The listing builds one solid part. Answer for the finished solid, in the listing's coordinates (mm). Give positions to 0.01 mm unless a question says otherwise; leave off trailing zeros. Loops run counter-clockwise (first coordinate to the right, second up) from the corner with the lowest first, then second, coordinate; pieces in that order, holes last. Notation, with made-up numbers: M 37,78 L 73,78 A15 cw 73,101 Z; hole C 70,-10 d11. An arc over 180 degrees is marked long. One line per item, written item: value. Start each with the question number.
Q1. A cutting plane is placed at B-B, the plane z = 9.5. Determine the outline of the cut face in (x, y), and give its area (3 significant figures).
Q2. Consider L1, parallel to Y at x = 1.25, z = 0; L2, parallel to Z at x = 0.2, y = 10; L3, parallel to Y at x = 0.3, z = -7. Determine where each line is inside the solid, lowest interval first.
Q3. A flat-ended cylindrical pin translates along its axis: pin 1 (5 mm diameter, centred on y = 95.25, z = 0, fed in from +X). Find the tip coordinate at first contact, or state that the pin passes through.
Q4. The mould has two halves that part along Z. Classify faces 1 (the cylindrical face through (0.783, 98.002, 1.755)), 2 (the cylindrical face through (0.78, 101.79, -4.5)), 3 (the flat face through (0, 45, 4)): +Z half, -Z half, draft (parallel to the pull), parting line (faces both ways), or undercut.
Q5. A cutting plane is placed at D-D, the plane y = 15. Determine the outline of the cut face in (x, z), and give its area (3 significant figures).
Q6. A cutting plane is placed at C-C, the plane x = 0.5. State how many separate pieces and enclosed holes the cut face has, and give its area (3 significant figures).
Q7. A cutting plane is placed at A-A, the plane z = 0. Determine the outline of the cut face in (x, y), and give its area (3 significant figures).
from build123d import *

# Parameters (mm, degrees)
SKETCH1_R               = 11.1125
BOSS_EXTRUDE1_DEPTH     = 1.5875
F_1_4_CLEARANCE_HOLE1_D = 6.5278
M8_CLEARANCE_HOLE1_D    = 8.4
BOSS_EXTRUDE2_DEPTH     = 1.5875


with BuildPart() as part:
    # Sketch1 → Boss-Extrude1 (new body)
    with BuildSketch(Plane(origin=(0, 0, 0), x_dir=(0, 0, -1), z_dir=(1, 0, 0))):
        with BuildLine():
            ThreePointArc((-26.033578217, 94.902839555), (-31.276267612, 90.601358567), (-32.328311992, 83.901975506))
            Line((-32.328311992, 83.901975506), (-25.778737426, 52.900096757))
            Line((-25.778737426, 52.900096757), (-24.225520946, 53.228235166))
            Line((-24.225520946, 53.228235166), (-18.975306409, 28.37677148))
            Line((-18.975306409, 28.37677148), (-20.528522889, 28.048633072))
            Line((-20.528522889, 28.048633072), (-13.978948323, -2.953245677))
            ThreePointArc((-13.978948323, -2.953245677), (1.957769706, -14.152730974), (14.255714644, 0.9525))
            Line((14.255714644, 0.9525), (11.936332499, 35.665833333))
            Line((11.936332499, 35.665833333), (10.352364205, 35.56))
            Line((10.352364205, 35.56), (8.655255319, 60.96))
            Line((8.655255319, 60.96), (10.239223613, 61.065833333))
            Line((10.239223613, 61.065833333), (7.919841469, 95.779166667))
            ThreePointArc((7.919841469, 95.779166667), (4.41923637, 101.843501055), (-2.520470923, 102.776694665))
            Line((-2.520470923, 102.776694665), (-5.244990973, 101.864332217))
            Line((-5.244990973, 101.864332217), (-4.740896788, 100.358993285))
            Line((-4.740896788, 100.358993285), (-22.804963983, 94.309863069))
            Line((-22.804963983, 94.309863069), (-23.309058168, 95.815202002))
            Line((-23.309058168, 95.815202002), (-26.033578217, 94.902839555))
        make_face()
        Circle(SKETCH1_R, mode=Mode.SUBTRACT)
    extrude(amount=BOSS_EXTRUDE1_DEPTH)

    # 1/4 Clearance Hole1 (through all)
    with Locations(Plane(origin=(1.5875, 0, 0), x_dir=(0, 0, -1), z_dir=(1, 0, 0))):
        with Locations((0, 95.25)):
            Hole(F_1_4_CLEARANCE_HOLE1_D / 2)

    # M8 Clearance Hole1 (through all)
    with Locations(Plane(origin=(1.5875, 0, 0), x_dir=(0, 0, -1), z_dir=(1, 0, 0))):
        with Locations((-23.00901311, 85.870805957)):
            Hole(M8_CLEARANCE_HOLE1_D / 2)

    # Sketch1<3> → Boss-Extrude2 (add)
    with BuildSketch(Plane(origin=(0, 0, 0), x_dir=(0, 0, -1), z_dir=(1, 0, 0))):
        Polygon((-5.244990973, 101.864332217), (-23.309058168, 95.815202002), (-22.804963983, 94.309863069), (-4.740896788, 100.358993285), align=None)
    extrude(amount=BOSS_EXTRUDE2_DEPTH)


solid = part.part
Answer block:
1. outline: M 0,-10.67 L 1.59,-10.67 L 1.59,-5.77 L 0,-5.77 Z; M 0,5.77 L 1.59,5.77 L 1.59,100.44 L 0,100.44 Z
1. area: 158 mm^2
2. L1: -14.29 to -11.11, 11.11 to 91.99, 98.51 to 103.19
2. L2: -13.65 to -4.85, 4.85 to 16.72
2. L3: -12.46 to -8.63, 8.63 to 98.99
3. pin 1: through
4. face 1: undercut
4. face 2: parting line
4. face 3: draft
5. outline: M 0,-13.32 L 1.59,-13.32 L 1.59,17.77 L 0,17.77 Z
5. area: 49.4 mm^2
6. separate pieces: 1
6. enclosed holes: 3
6. area: 3,300 mm^2
7. outline: M 0,-14.29 L 1.59,-14.29 L 1.59,-11.11 L 0,-11.11 Z; M 0,11.11 L 1.59,11.11 L 1.59,91.99 L 0,91.99 Z; M 0,98.51 L 1.59,98.51 L 1.59,103.19 L 0,103.19 Z
7. area: 141 mm^2
